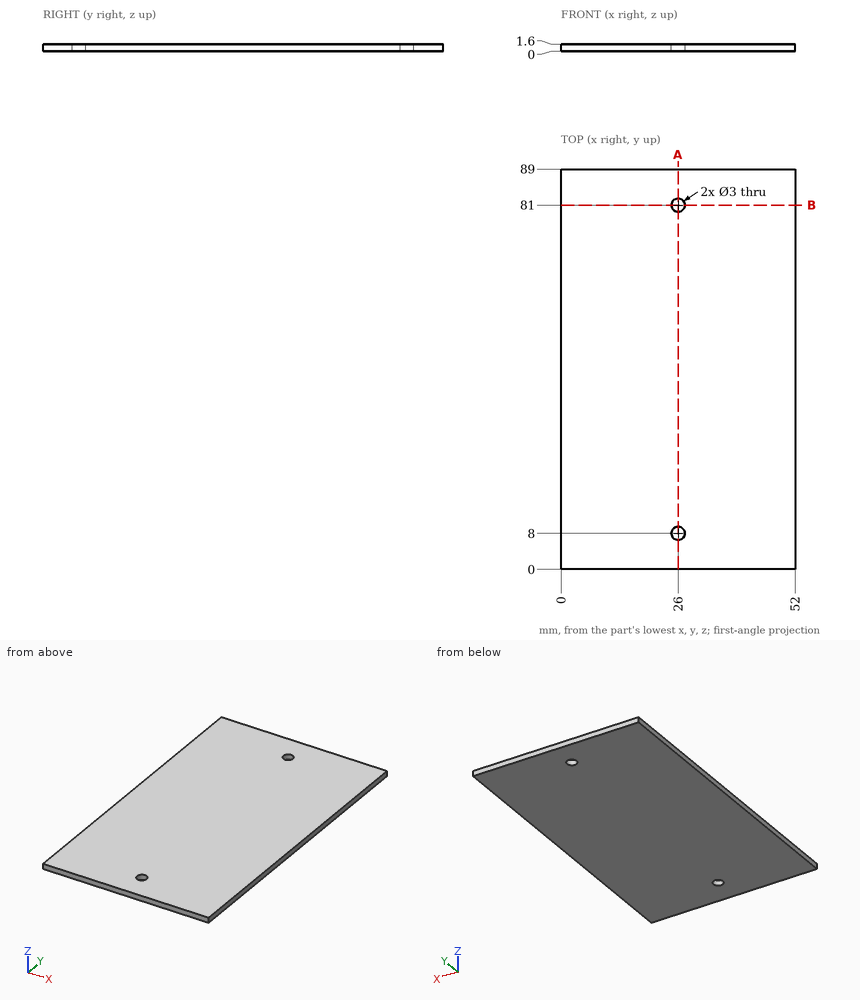
The figure shows three views and two pictorial views of one solid part (mm, origin at its lowest corner). Answer the questions. Coordinates: 2 decimals unless noted, no trailing zeros. Order: outer loops, then holes, each group sorted by start corner. A loop starts at its lowest first (then second) coordinate and runs counter-clockwise, first axis right, second up.
Q1. A cutting plane is placed at A-A, the plane x = 26. Write down the section's boundary in (y, z), and give its area (3 significant figures).
Q2. Consider line 1 (Y direction, x = 26, z = 1); line 2 (X direction, y = 8, z = 0.75). Determine where each line is inside the solid, lowest interval first.
Q3. A cutting plane is placed at B-B, the plane y = 81. Write down the section's boundary in (x, z), and give its area (3 significant figures).
Answers follow:
1. outline: (0, 0) - (6.5, 0) - (6.5, 1.6) - (0, 1.6) - close; (9.5, 0) - (79.5, 0) - (79.5, 1.6) - (9.5, 1.6) - close; (82.5, 0) - (89, 0) - (89, 1.6) - (82.5, 1.6) - close
1. area: 133 mm2
2. line 1: y = 0 to 6.5, 9.5 to 79.5, 82.5 to 89
2. line 2: x = 0 to 24.5, 27.5 to 52
3. outline: (0, 0) - (24.5, 0) - (24.5, 1.6) - (0, 1.6) - close; (27.5, 0) - (52, 0) - (52, 1.6) - (27.5, 1.6) - close
3. area: 78.4 mm2
